```python
from build123d import *

# Parameters (mm, degrees)
CUT_EXTRUDE_THIN1_DEPTH      = 52.961524227
CUT_EXTRUDE_THIN1_DEPTH_BACK = 52.961524227
SKETCH2_W                    = 30
SKETCH2_H                    = 44.72135955
CUT_EXTRUDE1_DEPTH           = 66.574385243
CUT_EXTRUDE1_DEPTH_BACK      = 12
SKETCH3_R                    = 6


with BuildPart() as part:
    # Sketch1 → Revolve1 (revolve)
    with BuildSketch(Plane.XY):
        with BuildLine():
            Line((0, 30), (0, -30))
            ThreePointArc((0, -30), (30, 0), (0, 30))
        make_face()
    revolve(axis=Axis((0, 30, 0), (0, -1, 0)))

    # Sketch2 → Cut-Extrude-Thin1 (cut, two sides: drawn at the far end of the back side and taken through both)
    with BuildSketch(Plane.XY.offset(-CUT_EXTRUDE_THIN1_DEPTH_BACK)):
        with Locations((35, 0)):
            Rectangle(SKETCH2_W, SKETCH2_H)
    extrude(amount=CUT_EXTRUDE_THIN1_DEPTH + CUT_EXTRUDE_THIN1_DEPTH_BACK, mode=Mode.SUBTRACT)

    # Sketch3 → Cut-Extrude1 (cut, two sides: drawn at the far end of the back side and taken through both)
    with BuildSketch(Plane(origin=(20, 0, 0), x_dir=(0, 0, -1), z_dir=(1, 0, 0)).offset(-CUT_EXTRUDE1_DEPTH_BACK)):
        with Locations(Location((0, 0, 0), (0, 0, 180))):
            Circle(SKETCH3_R)
    extrude(amount=CUT_EXTRUDE1_DEPTH + CUT_EXTRUDE1_DEPTH_BACK, mode=Mode.SUBTRACT)


solid = part.part
```
Check sheet for the modelled part. Datum: model origin and axes. Units: mm. Give positions to 0.01 mm unless a question says otherwise; leave off trailing zeros. Loops run counter-clockwise (first coordinate to the right, second up) from the corner with the lowest first, then second, coordinate; pieces in that order, holes last. Notation, with made-up numbers: M 68,3 L 102,3 A23 ccw 102,32 Z; hole C 56.25,33.25 d2. An arc over 180 degrees is marked long. Answer in a Markdown table with one row per item.
1) Cross-section at D-D (x = -14). Enter the section's corners in (y, z), plus the area to 3 significant figures.
Solutions:
| item | result |
|---|---|
| outline | C 0,0 d53.07 |
| area | 2,210 mm^2 |
2) Cross-section at A-A (y = 0). Enter the section's corners in (x, z), plus the area to 3 significant figures.
Solutions:
| item | result |
|---|---|
| outline | M 8,-6 L 8,6 L 20,6 L 20,22.36 A30 ccw long 20,-22.36 L 20,-6 Z |
| area | 2,370 mm^2 |
3) Cross-section at B-B (z = -4). Enter the section's corners in (x, y), plus the area to 3 significant figures.
Solutions:
| item | result |
|---|---|
| outline | M 8,-4.47 L 8,4.47 L 20,4.47 L 20,22 A29.73 ccw long 20,-22 L 20,-4.47 Z |
| area | 2,370 mm^2 |
4) Depth check by flat-ended pin: pin 1 (4 mm diameter, centred on x = 8, z = 21, fed in from +Y); pin 2 (7 mm diameter, centred on y = 0, z = 0, fed in from -X); pin 3 (1 mm diameter, centred on y = 5, z = 23, fed in from -X). Enter the tip coordinate at first touch or a pass-through.
Solutions:
| item | result |
|---|---|
| pin 1 | stops at y = 21.93 |
| pin 2 | stops at x = -30 |
| pin 3 | stops at x = -19.22 |
5) Thickness scan on line 1 (Y direction, x = 12.5, z = 0); line 2 (Y direction, x = 11, z = 0); line 3 (Z direction, x = 11, y = 1). Record the ranges inside material, lowest first.
Solutions:
| item | result |
|---|---|
| line 1 | y = -27.27 to -6, 6 to 27.27 |
| line 2 | y = -27.91 to -6, 6 to 27.91 |
| line 3 | z = -27.89 to -5.92, 5.92 to 27.89 |
6) Cross-section at C-C (x = 15.5). Enter the section's corners in (y, z), plus the area to 3 significant figures.
Solutions:
| item | result |
|---|---|
| outline | C 0,0 d51.37; hole C 0,0 d12 |
| area | 1,960 mm^2 |
7) Mould release check, pull along Z, two halves, no side actions. Record for faces 1 (the face through (20, 5, 5)), 2 (the face through (8, 0, 0)): released by +Z, released by -Z, zero draft, split by the parting line, or undercut.
Solutions:
| item | result |
|---|---|
| face 1 | zero draft |
| face 2 | undercut |
